Build history of the part. All positions in model axes, mm. Face numbers are marked on the shaded views. A direction names the side the tool comes from. Give positions to 0.01 mm unless a question says otherwise; leave off trailing zeros. Order: outer loops, then holes, each group sorted by start corner. A loop starts at its lowest first (then second) coordinate and runs counter-clockwise, first axis right, second up. Notation, with made-up numbers: M 34.25,40.25 L 62.25,40.25 A12 ccw 62.25,44.25 Z; hole C -17.75,45 d9. An arc over 180 degrees is marked long. Answer as CSV lines item,"result".
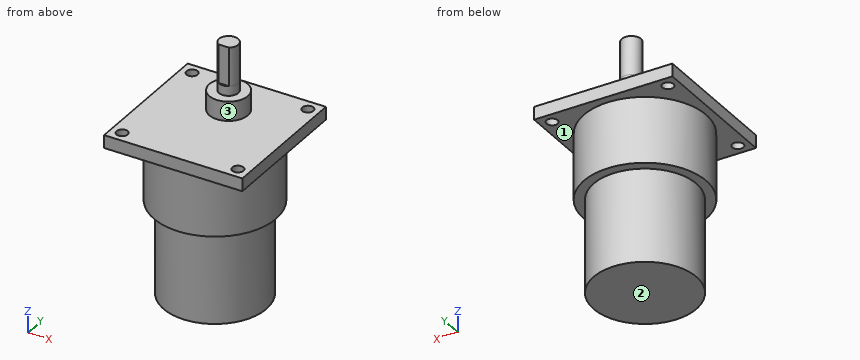
from build123d import *

# Parameters (mm, degrees)
SKETCH_W     = 43
SKETCH_H     = 43
PAD_DEPTH    = 4
SKETCH001_R  = 1.75
POCKET_DEPTH = 4
SKETCH002_R  = 6
PAD001_DEPTH = 6
SKETCH003_R  = 3
PAD002_DEPTH = 3
PAD003_DEPTH = 12
SKETCH005_R  = 19
PAD004_DEPTH = 20.5
SKETCH006_R  = 16
PAD005_DEPTH = 29


with BuildPart() as part:
    # Sketch → Pad (new body)
    with BuildSketch(Plane.XY):
        Rectangle(SKETCH_W, SKETCH_H)
    extrude(amount=PAD_DEPTH)

    # Sketch001 (on Face6 of Pad) → Pocket (cut)
    with BuildSketch(Plane.XY.offset(4)):
        with Locations((-18, 18)):
            Circle(SKETCH001_R)
        with Locations((18, 18)):
            Circle(SKETCH001_R)
        with Locations((18, -18)):
            Circle(SKETCH001_R)
        with Locations((-18, -18)):
            Circle(SKETCH001_R)
    extrude(amount=-POCKET_DEPTH, mode=Mode.SUBTRACT)

    # Sketch002 (on Face5 of Pocket) → Pad001 (join)
    with BuildSketch(Plane.XY.offset(4)):
        with Locations((0, 7)):
            Circle(SKETCH002_R)
    extrude(amount=PAD001_DEPTH)

    # Sketch003 (on Face12 of Pad001) → Pad002 (join)
    with BuildSketch(Plane.XY.offset(10)):
        with Locations((0, 7)):
            Circle(SKETCH003_R)
    extrude(amount=PAD002_DEPTH)

    # Sketch004 (on Face14 of Pad002) → Pad003 (join)
    with BuildSketch(Plane.XY.offset(13)):
        with BuildLine():
            ThreePointArc((1.658312, 4.5), (0, 10), (-1.658312, 4.5))
            Line((-1.658312, 4.5), (1.658312, 4.5))
        make_face()
    extrude(amount=PAD003_DEPTH)

    # Sketch005 (on Face4 of Pad003) → Pad004 (join)
    with BuildSketch(Plane(origin=(0, 0, 0), x_dir=(1, 0, 0), z_dir=(0, 0, -1))):
        Circle(SKETCH005_R)
    extrude(amount=PAD004_DEPTH)

    # Sketch006 (on Face13 of Pad004) → Pad005 (join)
    with BuildSketch(Plane(origin=(0, 0, -20.5), x_dir=(1, 0, 0), z_dir=(0, 0, -1))):
        Circle(SKETCH006_R)
    extrude(amount=PAD005_DEPTH)


solid = part.part
Item 1: 3-axis set-ups, long thin cutter, end or side, ignore diameter. For the marked faces 1, 2 and 3: which of +Z, -Z, +X, -X, +Y, -Y reach the whole face in a straight line?
Geometry says:
face 1,"-Z"
face 2,"-Z, +X, -X, +Y, -Y"
face 3,"+Z"
Item 2: Band-saw the part on B-B (x = -12.5). Give the cut face in (y, z).
Geometry says:
outline,"M -21.5,0 L -14.31,0 L -14.31,-20.5 L -9.99,-20.5 L -9.99,-49.5 L 9.99,-49.5 L 9.99,-20.5 L 14.31,-20.5 L 14.31,0 L 21.5,0 L 21.5,4 L -21.5,4 Z"
Item 3: Drop flat-ended pins along their axis: pin 1 (3 mm diameter, centred on x = 18, y = -18, fed in from +Z); pin 2 (10 mm diameter, centred on x = 5.5, y = -8.5, fed in from +Z); pin 3 (4.5 mm diameter, centred on x = -18, y = -18, fed in from -Z); pin 4 (3 mm diameter, centred on x = 14.5, z = -18.5, fed in from +Y). Give the stop position or say it passes through.
Geometry says:
pin 1,"passes through"
pin 2,"stops at z = 4"
pin 3,"stops at z = 0"
pin 4,"stops at y = 13.86"
Item 4: Probe line 1 along Y through (x, z) = (-18, 2); line 2 along Z through (x, y) = (18.5, 7.5); line 3 along Z through (x, y) = (-5.5, -4). List the from-to ranges inside material, lowest first. Write a range as from..to.
Geometry says:
line 1,"y = -21.5..-19.75, -16.25..16.25, 19.75..21.5"
line 2,"z = 0..4"
line 3,"z = -49.5..4"
Item 5: Band-saw the part on A-A (y = 0). Give the cut face in (x, z).
Geometry says:
outline,"M -21.5,0 L -19,0 L -19,-20.5 L -16,-20.5 L -16,-49.5 L 16,-49.5 L 16,-20.5 L 19,-20.5 L 19,0 L 21.5,0 L 21.5,4 L -21.5,4 Z"
Item 6: Band-saw the part on C-C (y = 18). Give the cut face in (x, z).
Geometry says:
outline,"M -21.5,0 L -19.75,0 L -19.75,4 L -21.5,4 Z; M -16.25,0 L -6.08,0 L -6.08,-20.5 L 6.08,-20.5 L 6.08,0 L 16.25,0 L 16.25,4 L -16.25,4 Z; M 19.75,0 L 21.5,0 L 21.5,4 L 19.75,4 Z"
